Geometry check sheet. Reference: the model listing, model coordinates, mm. Face numbers are marked on the shaded views. Round coordinates to 2 decimals unless told otherwise and drop trailing zeros. Order: outer loops, then holes, each group sorted by start corner. A loop starts at its lowest first (then second) coordinate and runs counter-clockwise, first axis right, second up.
(1) Draft check along Y on the marked faces 1, 2, 3 and 4. Enter one of: pulls with the +Y half, pulls with the -Y half, needs draft (parallel to the pull), parting line crosses it, or undercut.
(2) Cross-section at B-B on y = -17.5. Enter the section's corners in (x, z) (3 decimals), and give its area (3 significant figures).
(3) Cross-section at A-A on x = 9. Enter the section's corners in (y, z) (3 decimals).
(4) Thickness scan on L1, parallel to Y at x = -1, z = 1.25 (3 decimals); L2, parallel to Y at x = -18, z = 2.5 (3 decimals); L3, parallel to X at y = -29, z = 2.75 (3 decimals). Record the ranges inside material, lowest first.
(5) Cross-section at C-C on x = -21.5. Enter the section's corners in (y, z) (3 decimals), and give its area (3 significant figures).
(6) Gauge pin test, flat end, axial feed: P1, Ø1, axis at x = -3.5, y = 20.5, coming from the +Z side (3 decimals). Record the tip position at first contact, or that the pin passes through.
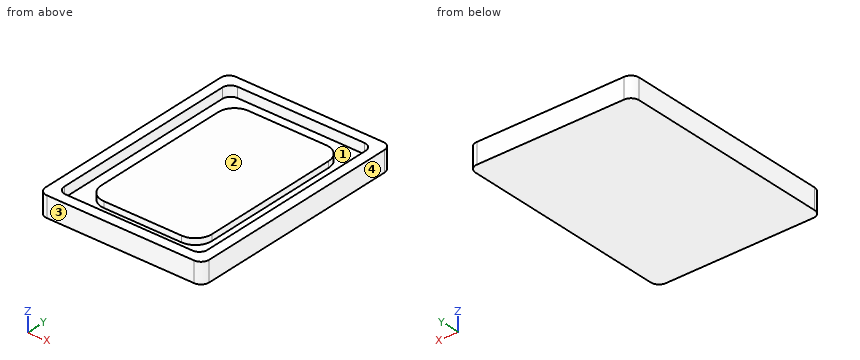
from build123d import *

# Parameters (mm, degrees)
F0_W     = 50.8
F0_H     = 69.85
F1_DEPTH = 3.175
F2_R     = 2.54
F3_W     = 44.45
F3_H     = 63.5
F4_DEPTH = 3.175
F5_R     = 2.54
F7_DEPTH = 1.905


with BuildPart() as f1:
    # F0 (on Top) → F1 (new body, symmetric)
    with BuildSketch(Plane.XY):
        Rectangle(F0_W, F0_H)
    extrude(amount=F1_DEPTH, both=True)

    # F2
    f2_edges = [f1.edges().sort_by_distance(p)[0] for p in [
        (25.4, -34.925, 0),
        (-25.4, -34.925, 0),
        (25.4, 34.925, 0),
        (-25.4, 34.925, 0),
    ]]
    fillet(f2_edges, radius=F2_R)

    # F3 (on face) → F4 (cut)
    with BuildSketch(Plane.XY.offset(3.175)):
        Rectangle(F3_W, F3_H)
    extrude(amount=-F4_DEPTH, mode=Mode.SUBTRACT)

    # F5
    f5_edges = [f1.edges().sort_by_distance(p)[0] for p in [
        (-22.225, 31.75, 1.5875),
        (22.225, 31.75, 1.5875),
        (-22.225, -31.75, 1.5875),
        (22.225, -31.75, 1.5875),
    ]]
    fillet(f5_edges, radius=F5_R)

    # F6 (on face) → F7 (join)
    with BuildSketch(Plane.XY):
        with BuildLine():
            ThreePointArc((-17.145, -21.59), (-15.657102, -25.182102), (-12.065, -26.67))
            Line((-12.065, -26.67), (12.065, -26.67))
            ThreePointArc((12.065, -26.67), (15.657102, -25.182102), (17.145, -21.59))
            Line((17.145, -21.59), (17.145, 21.59))
            ThreePointArc((17.145, 21.59), (15.657102, 25.182102), (12.065, 26.67))
            Line((12.065, 26.67), (-12.065, 26.67))
            ThreePointArc((-12.065, 26.67), (-15.657102, 25.182102), (-17.145, 21.59))
            Line((-17.145, 21.59), (-17.145, -21.59))
        make_face()
    extrude(amount=F7_DEPTH)


solid = f1.part
Found:
1. face 1: undercut
1. face 2: undercut
1. face 3: pulls with the -Y half
1. face 4: needs draft
2. outline: (-25.4, -3.175) - (25.4, -3.175) - (25.4, 3.175) - (22.225, 3.175) - (22.225, 0) - (17.145, 0) - (17.145, 1.905) - (-17.145, 1.905) - (-17.145, 0) - (-22.225, 0) - (-22.225, 3.175) - (-25.4, 3.175) - close
2. area: 247 mm2
3. outline: (-34.925, -3.175) - (34.925, -3.175) - (34.925, 3.175) - (31.75, 3.175) - (31.75, 0) - (26.67, 0) - (26.67, 1.905) - (-26.67, 1.905) - (-26.67, 0) - (-31.75, 0) - (-31.75, 3.175) - (-34.925, 3.175) - close
4. L1: y = -34.925 to -31.75, -26.67 to 26.67, 31.75 to 34.925
4. L2: y = -34.925 to -31.75, 31.75 to 34.925
4. L3: x = -25.4 to -22.225, 22.225 to 25.4
5. outline: (-34.925, -3.175) - (34.925, -3.175) - (34.925, 3.175) - (30.987, 3.175) - (30.987, 0) - (-30.987, 0) - (-30.987, 3.175) - (-34.925, 3.175) - close
5. area: 247 mm2
6. P1: stops at z = 1.905
